For this review, take the finished solid that the model builds, in its own axes (mm). Face numbers are marked on the shaded views. Coordinates: 2 decimals unless noted, no trailing zeros. Order: outer loops, then holes, each group sorted by start corner. A loop starts at its lowest first (then second) coordinate and runs counter-clockwise, first axis right, second up. Notation, with made-up numbers: (-18, 23.5) -> (2, 23.5) arc R25 cw to (2, 58.5) -> close; hole circle Ø10 at (69.25, 13). An arc over 180 degrees is marked (long way). Return JSON: item names as keys, results as strings. Group by question number.
Item 1: Insertion check: pin 1 (9 mm diameter, centred on x = 0, y = 0, fed in from +Z); pin 2 (0.9 mm diameter, centred on x = 31.5, z = 1, fed in from +Y); pin 3 (1.5 mm diameter, centred on x = 12.5, z = 0.5, fed in from -Y). Each pin has a flat end and moves straight along its axis. Give the tip position at first contact, or say it passes through.
Item 2: Draft analysis for pull direction Y (two halves, no side actions). For the marked faces 1, 2 and 3, state which applies: +Y half, -Y half, draft (parallel to the pull), parting line (faces both ways), or undercut.
Item 3: Take a section at B-B (z = 0.5). Write out the cut boundary in (x, y).
Item 4: For line 1 along Y through (x, z) = (0, 2); line 2 along Y through (x, z) = (-1, 2.55); line 3 along Y through (x, z) = (21, 0.8), list the stretches that pass through material, from the lowest coordinate up.
Item 5: Take a section at A-A (x = 0). Write out the cut boundary in (y, z).
Item 6: Take a section at C-C (y = 7.2). Write out the cut boundary in (x, z).
```python
from build123d import *

# Parameters (mm, degrees)
ESBO_O1_R                = 1.55
RESSALTO_EXTRUS_O1_DEPTH = 3


with BuildPart() as part:
    # Esbo_o1 → Ressalto-extrus_o1 (new body)
    # profile 1 of 3: a face of its own
    with BuildSketch(Plane.XY):
        with BuildLine():
            Line((2.872281323, 2), (10.816653826, 2))
            ThreePointArc((10.816653826, 2), (-11, 0), (10.816653826, -2))
            Line((10.816653826, -2), (2.872281323, -2))
            ThreePointArc((2.872281323, -2), (-3.5, 0), (2.872281323, 2))
        make_face()
        with Locations((0, -7.199999987)):
            Circle(ESBO_O1_R, mode=Mode.SUBTRACT)
        with Locations((-7.199999991, 0)):
            Circle(ESBO_O1_R, mode=Mode.SUBTRACT)
        with Locations((0, 7.199999994)):
            Circle(ESBO_O1_R, mode=Mode.SUBTRACT)
    # profile 2 of 3: a face of its own
    with BuildSketch(Plane.XY):
        with BuildLine():
            Line((40, -2), (40, 0))
            Line((40, 0), (40, 2))
            Line((40, 2), (10.816653826, 2))
            ThreePointArc((10.816653826, 2), (10.954067557, 1.004193186), (11, 0))
            ThreePointArc((11, 0), (10.954067557, -1.004193186), (10.816653826, -2))
            Line((10.816653826, -2), (40, -2))
        make_face()
    # profile 3 of 3: a face of its own
    with BuildSketch(Plane.XY):
        with BuildLine():
            ThreePointArc((11, 0), (10.954067557, 1.004193186), (10.816653826, 2))
            Line((10.816653826, 2), (2.872281323, 2))
            ThreePointArc((2.872281323, 2), (3.339385021, 1.048097173), (3.5, 0))
            ThreePointArc((3.5, 0), (3.339385021, -1.048097173), (2.872281323, -2))
            Line((2.872281323, -2), (10.816653826, -2))
            ThreePointArc((10.816653826, -2), (10.954067557, -1.004193186), (11, 0))
        make_face()
    extrude(amount=RESSALTO_EXTRUS_O1_DEPTH)


solid = part.part
```
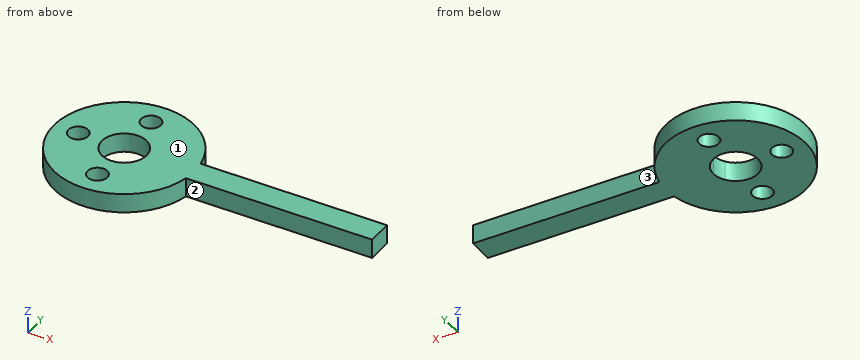
Findings below:
{
 "1": {"pin 1": "stops at z = 3", "pin 2": "stops at y = 2", "pin 3": "stops at y = -2"},
 "2": {"face 1": "draft", "face 2": "-Y half", "face 3": "+Y half"},
 "3": {"outline": "(10.82, -2) -> (40, -2) -> (40, 2) -> (10.82, 2) arc R11 ccw (long way) to start; hole circle Ø3.1 at (-7.2, 0); hole circle Ø7 at (0, 0); hole circle Ø3.1 at (0, -7.2); hole circle Ø3.1 at (0, 7.2)"},
 "4": {"line 1": "y = -11 to -8.75, -5.65 to -3.5, 3.5 to 5.65, 8.75 to 11", "line 2": "y = -10.95 to -8.38, -6.02 to -3.35, 3.35 to 6.02, 8.38 to 10.95", "line 3": "y = -2 to 2"},
 "5": {"outline": "(-11, 0) -> (-8.75, 0) -> (-8.75, 3) -> (-11, 3) -> close; (-5.65, 0) -> (-3.5, 0) -> (-3.5, 3) -> (-5.65, 3) -> close; (3.5, 0) -> (5.65, 0) -> (5.65, 3) -> (3.5, 3) -> close; (8.75, 0) -> (11, 0) -> (11, 3) -> (8.75, 3) -> close"},
 "6": {"outline": "(-8.32, 0) -> (-1.55, 0) -> (-1.55, 3) -> (-8.32, 3) -> close; (1.55, 0) -> (8.32, 0) -> (8.32, 3) -> (1.55, 3) -> close"}
}
